Can you work these out from the model? Positions are in its coordinate system, mm. A direction names the side the tool comes from. Coordinates: 2 decimals unless noted, no trailing zeros. Loops run counter-clockwise (first coordinate to the right, second up) from the corner with the lowest first, then second, coordinate; pieces in that order, holes last.
```python
from build123d import *

# Parameters (mm, degrees)
SKETCH1_W           = 9.906
SKETCH1_H           = 8.128
BOSS_EXTRUDE1_DEPTH = 4.318
SKETCH2_W           = 9.906
SKETCH2_H           = 6.401
SKETCH2_R           = 1.778
BOSS_EXTRUDE3_DEPTH = 1.219
BOSS_EXTRUDE4_DEPTH = 13.284


with BuildPart() as part:
    # Sketch1 → Boss-Extrude1 (new body)
    with BuildSketch(Plane(origin=(0, 0, 0), x_dir=(0, 0, -1), z_dir=(1, 0, 0))):
        Rectangle(SKETCH1_W, SKETCH1_H)
    extrude(amount=BOSS_EXTRUDE1_DEPTH)

    # Sketch2 → Boss-Extrude3 (add)
    with BuildSketch(Plane(origin=(0, 0, 0), x_dir=(0, 0, -1), z_dir=(1, 0, 0))):
        with Locations((0, 7.2645)):
            Rectangle(SKETCH2_W, SKETCH2_H)
        with Locations((0, 7.798)):
            Circle(SKETCH2_R, mode=Mode.SUBTRACT)
    extrude(amount=BOSS_EXTRUDE3_DEPTH)

    # Sketch3 → Boss-Extrude4 (add)
    with BuildSketch(Plane(origin=(0, -4.064, 0), x_dir=(-1, 0, 0), z_dir=(0, -1, 0))):
        Polygon((-2.591, -1.949316438), (-2.591, -1.314316438), (-2.21, -1.314316438), (-2.21, -1.631816438), (-2.21, -1.949316438), align=None)
        Polygon((-2.21, 0.068183562), (-2.21, -0.249316438), (-2.591, -0.249316438), (-2.591, 0.385683562), (-2.21, 0.385683562), align=None)
        Polygon((-2.591, -3.649316438), (-2.591, -3.014316438), (-2.21, -3.014316438), (-2.21, -3.331816438), (-2.21, -3.649316438), align=None)
        Polygon((-2.591, 1.450683562), (-2.591, 2.085683562), (-2.21, 2.085683562), (-2.21, 1.768183562), (-2.21, 1.450683562), align=None)
        Polygon((-2.591, 3.150683562), (-2.591, 3.785683562), (-2.21, 3.785683562), (-2.21, 3.468183562), (-2.21, 3.150683562), align=None)
    extrude(amount=BOSS_EXTRUDE4_DEPTH)


solid = part.part
```
Item 1: Suppose I cut it at A-A, the plane y = -6. Please give me the cut outline in (x, z).
Results are:
outline: (2.21, -3.79) - (2.59, -3.79) - (2.59, -3.15) - (2.21, -3.15) - close; (2.21, -2.09) - (2.59, -2.09) - (2.59, -1.45) - (2.21, -1.45) - close; (2.21, -0.39) - (2.59, -0.39) - (2.59, 0.25) - (2.21, 0.25) - close; (2.21, 1.31) - (2.59, 1.31) - (2.59, 1.95) - (2.21, 1.95) - close; (2.21, 3.01) - (2.59, 3.01) - (2.59, 3.65) - (2.21, 3.65) - close
Item 2: Suppose I cut it at B-B, the plane z = 0. Please give me the cut outline in (x, y) (3 decimals).
Results are:
outline: (0, -4.064) - (2.21, -4.064) - (2.21, -17.348) - (2.591, -17.348) - (2.591, -4.064) - (4.318, -4.064) - (4.318, 4.064) - (1.219, 4.064) - (1.219, 6.02) - (0, 6.02) - close; (0, 9.576) - (1.219, 9.576) - (1.219, 10.465) - (0, 10.465) - close
Item 3: On a 3-axis mill with a long thin cutter (end or side, diameter ignored), from which of +Z, -Z, +X, -X, +Y, -Y can I reach the whole of each face in a straight line? I mean faces 4 (the face through (4.318, 0, 0)), 5 (the face through (1.219, 6, 1)). Say none if no direction works.
Results are:
face 4: +Z, -Z, +X, +Y, -Y
face 5: +Z, -Z, +X, +Y
Item 4: I need wall thicknesses on line 1 along Y through (x, z) = (0.7, 0) (3 decimals); line 2 along Y through (x, z) = (3.5, 2); line 3 along X through (y, z) = (9.25, -2.5). Which ranges of each line are inside material? Lowest first, please.
Results are:
line 1: y = -4.064 to 6.02, 9.576 to 10.465
line 2: y = -4.06 to 4.06
line 3: x = 0 to 1.22
Item 5: Suppose I cut it at C-C, the plane x = 0.3. Please give me the cut outline in (y, z) (3 decimals), plus the area to 3 significant figures.
Results are:
outline: (-4.064, -4.953) - (10.465, -4.953) - (10.465, 4.953) - (-4.064, 4.953) - close; hole circle Ø3.556 at (7.798, 0)
area: 134 mm2
Item 6: I'm going to push flat-ended pins straight in: P1, Ø1, axis at x = 1.5, z = -0.5, coming from the -Y side; P2, Ø3, axis at y = -10.5, z = -1.5, coming from the +X side; P3, Ø2, axis at x = 3.5, z = -1.5, coming from the +Y side. Where does each tip first touch, or does it pass through?
Results are:
P1: stops at y = -4.06
P2: stops at x = 2.59
P3: stops at y = 4.06
Item 7: Suppose I cut it at D-D, the plane z = -4.5. Please give me the cut outline in (x, y) (3 decimals), plus the area to 3 significant figures.
Results are:
outline: (0, -4.064) - (4.318, -4.064) - (4.318, 4.064) - (1.219, 4.064) - (1.219, 10.465) - (0, 10.465) - close
area: 42.9 mm2
Item 8: We'd pull the mould along Y, two halves only. Please class faces 1 (the face through (0.601, 7.876, 1.776)), 2 (the face through (3, 4.064, 0)), 3 (the face through (0, 3, 0)): +Y half, -Y half, draft (parallel to the pull), parting line (faces both ways), or undercut.
Results are:
face 1: undercut
face 2: +Y half
face 3: draft
